The drawing under review shows one solid part. Ordinate dimensions are in mm from its lowest x, y, z. Give positions to 0.01 mm unless a question says otherwise; leave off trailing zeros. Write each loop counter-clockwise with the first axis right and the second up, starting at its lowest first coordinate (ties: lowest second). Pieces come first, ordered by that corner, then holes.
Q1. Insertion check: P1, Ø1, axis at y = 37, z = 1, coming from the -X side. The pin has a flat end and moves straight along its axis. Give the tip position at first contact, or say it passes through.
Q2. We need section A-A (x = 24). Write out the cut boundary in (y, z).
Q3. We need section D-D (y = 44). Write out the cut boundary in (x, z).
Q4. We need section C-C (z = 0.3). Give the number of separate pieces and of enclosed holes in the cut face, then the cut area to 3 significant figures.
Q5. We need section B-B (y = 24). Write out the cut boundary in (x, z).
Q6. For line 1 (Y direction, x = 24, z = 0.7); line 2 (X direction, y = 25, z = 0.85); line 3 (X direction, y = 34, z = 0.9), list the stretches that pass through material, from the lowest coordinate up.
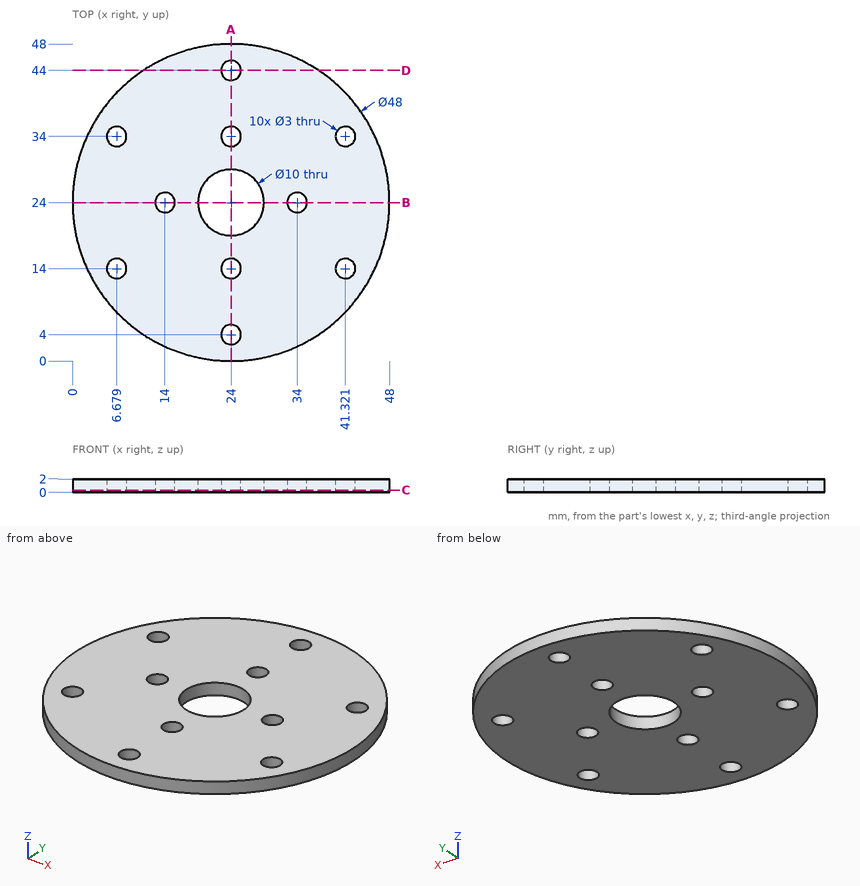
Computed:
1. P1: stops at x = 3.51
2. outline: (0, 0) - (2.5, 0) - (2.5, 2) - (0, 2) - close; (5.5, 0) - (12.5, 0) - (12.5, 2) - (5.5, 2) - close; (15.5, 0) - (19, 0) - (19, 2) - (15.5, 2) - close; (29, 0) - (32.5, 0) - (32.5, 2) - (29, 2) - close; (35.5, 0) - (42.5, 0) - (42.5, 2) - (35.5, 2) - close; (45.5, 0) - (48, 0) - (48, 2) - (45.5, 2) - close
3. outline: (10.73, 0) - (22.5, 0) - (22.5, 2) - (10.73, 2) - close; (25.5, 0) - (37.27, 0) - (37.27, 2) - (25.5, 2) - close
4. separate pieces: 1
4. enclosed holes: 11
4. area: 1,660 mm2
5. outline: (0, 0) - (12.5, 0) - (12.5, 2) - (0, 2) - close; (15.5, 0) - (19, 0) - (19, 2) - (15.5, 2) - close; (29, 0) - (32.5, 0) - (32.5, 2) - (29, 2) - close; (35.5, 0) - (48, 0) - (48, 2) - (35.5, 2) - close
6. line 1: y = 0 to 2.5, 5.5 to 12.5, 15.5 to 19, 29 to 32.5, 35.5 to 42.5, 45.5 to 48
6. line 2: x = 0.02 to 12.88, 15.12 to 19.1, 28.9 to 32.88, 35.12 to 47.98
6. line 3: x = 2.18 to 5.18, 8.18 to 22.5, 25.5 to 39.82, 42.82 to 45.82
